Design review of the part built by this model. Coordinates are the model's own, in mm. Give positions to 0.01 mm unless a question says otherwise; leave off trailing zeros. Write each loop counter-clockwise with the first axis right and the second up, starting at its lowest first coordinate (ties: lowest second). Pieces come first, ordered by that corner, then holes. Notation, with made-up numbers: M -15,-37.75 L 42,-37.75 A14 cw 42,-30.75 Z; hole C 2,47.25 d5. An arc over 180 degrees is marked long. Use one line per item in the form item = value. Start each with the question number.
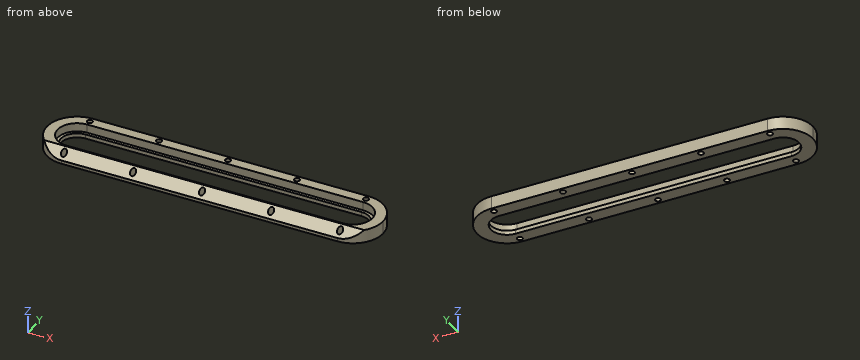
from build123d import *

# Parameters (mm, degrees)
SKETCH1_W              = 247.65
SKETCH1_H              = 44.45
BOSS_EXTRUDE1_DEPTH    = 9.525
CUT_EXTRUDE1_DEPTH     = 6.35
CUT_EXTRUDE3_DEPTH     = 126.963898598
CUT_EXTRUDE2_DEPTH     = 127.163809688
F_10_32_TAPPED_HOLE1_D = 4.0386
CHAMFER2_SIZE          = 6.985


with BuildPart() as part:
    # Sketch1 → Boss-Extrude1 (new body)
    with BuildSketch(Plane.XY):
        Rectangle(SKETCH1_W, SKETCH1_H)
    extrude(amount=BOSS_EXTRUDE1_DEPTH)

    # Sketch2 → Cut-Extrude1 (cut)
    with BuildSketch(Plane.XY.offset(9.525)):
        with BuildLine():
            Line((101.6, -14.351), (-101.6, -14.351))
            ThreePointArc((-101.6, -14.351), (-115.951, 0), (-101.6, 14.351))
            Line((-101.6, 14.351), (101.6, 14.351))
            ThreePointArc((101.6, 14.351), (115.951, 0), (101.6, -14.351))
        make_face()
    extrude(amount=-CUT_EXTRUDE1_DEPTH, mode=Mode.SUBTRACT)

    # Sketch14 → Cut-Extrude3 (cut, through all)
    with BuildSketch(Plane.XY.offset(3.175)):
        with BuildLine():
            Line((101.6, 11.96975), (-101.6, 11.96975))
            ThreePointArc((-101.6, 11.96975), (-113.56975, 0), (-101.6, -11.96975))
            Line((-101.6, -11.96975), (101.6, -11.96975))
            ThreePointArc((101.6, -11.96975), (113.56975, 0), (101.6, 11.96975))
        make_face()
    extrude(amount=-CUT_EXTRUDE3_DEPTH, mode=Mode.SUBTRACT)

    # Sketch3 → Cut-Extrude2 (cut, through all)
    with BuildSketch(Plane.XY.offset(9.525)):
        with BuildLine():
            ThreePointArc((-123.825, -1.74e-07), (-117.315448274, 15.71544815), (-101.6, 22.225))
            Line((-101.6, 22.225), (-123.825, 22.225))
            Line((-123.825, 22.225), (-123.825, -1.74e-07))
        make_face()
        with BuildLine():
            ThreePointArc((-101.6, -22.225), (-117.31544815, -15.715448274), (-123.825, -1.74e-07))
            Line((-123.825, -1.74e-07), (-123.825, -22.225))
            Line((-123.825, -22.225), (-101.6, -22.225))
        make_face()
        with BuildLine():
            Line((123.825, -22.225), (123.825, -6.4e-08))
            ThreePointArc((123.825, -6.4e-08), (117.315448189, -15.715448235), (101.6, -22.225))
            Line((101.6, -22.225), (123.825, -22.225))
        make_face()
        with BuildLine():
            Line((123.825, 22.225), (101.6, 22.225))
            ThreePointArc((101.6, 22.225), (117.315448235, 15.715448189), (123.825, -6.4e-08))
            Line((123.825, -6.4e-08), (123.825, 22.225))
        make_face()
    extrude(amount=-CUT_EXTRUDE2_DEPTH, mode=Mode.SUBTRACT)

    # #10-32 Tapped Hole1 (through all)
    with Locations(Plane.XY.offset(9.525)):
        with Locations((-101.6, 18.415), (-50.8, 18.415), (0, 18.415), (50.8, 18.415), (101.6, 18.415), (101.6, -18.415), (50.8, -18.415), (0, -18.415), (-50.8, -18.415), (-101.6, -18.415)):
            Hole(F_10_32_TAPPED_HOLE1_D / 2)

    # Chamfer2
    # the kernel refuses this chamfer: 6.985 mm, written as the material it takes off along each edge
    with BuildSketch(Plane(origin=(-119.563205671, -22.225, 9.525), x_dir=(0, 0.9996219169112968, 0.027495876610586303), z_dir=(1, 0, 0))) as chamfer2_piece_1:
        Polygon((CHAMFER2_SIZE * 0.999621916911, -CHAMFER2_SIZE * 0.0274958766106), (-CHAMFER2_SIZE * 0.0274958766106, -CHAMFER2_SIZE * 0.999621916911), (0, 0), align=None)
    extrude(amount=239.126411342, mode=Mode.SUBTRACT)


solid = part.part
1. We need section C-C (x = 108.5). State the section outline as (y, z) points (3 decimals).
2. We need section A-A (x = 15.5). State the section outline as (y, z) points (3 decimals).
3. We need section B-B (x = 50.8). State the section outline as (y, z) points (3 decimals).
4. Clearance check with flat-ended pins moving along their axes: pin 1 Ø1 at (y, z) = (2, 2.5) entering from +X; pin 2 Ø1 at (x, z) = (-69, 4) entering from -Y (3 decimals); pin 3 Ø4 at (y, z) = (-3.5, 7.5) entering from -X. State where each tip first meets the part, or that it passes through.
5. To check wall thickness, follow L1, parallel to Y at x = -50.8, z = 7.5 (3 decimals); L2, parallel to Y at x = 49.5, z = 6 (3 decimals); L3, parallel to X at y = 19, z = 2. State the ranges of each line that lie inside material, in increasing order.
Answer block:
q1.outline = M -21.127,0 L -9.781,0 L -9.781,3.175 L -12.583,3.175 L -12.583,9.525 L -15.24,9.525 L -21.127,3.638 Z; M 9.781,0 L 21.127,0 L 21.127,9.525 L 12.583,9.525 L 12.583,3.175 L 9.781,3.175 Z
q2.outline = M -22.225,0 L -11.97,0 L -11.97,3.175 L -14.351,3.175 L -14.351,9.525 L -15.24,9.525 L -22.225,2.54 Z; M 11.97,0 L 22.225,0 L 22.225,9.525 L 14.351,9.525 L 14.351,3.175 L 11.97,3.175 Z
q3.outline = M -22.225,0 L -20.434,0 L -20.434,4.331 L -22.225,2.54 Z; M -16.396,0 L -11.97,0 L -11.97,3.175 L -14.351,3.175 L -14.351,9.525 L -15.24,9.525 L -16.396,8.369 Z; M 11.97,0 L 16.396,0 L 16.396,9.525 L 14.351,9.525 L 14.351,3.175 L 11.97,3.175 Z; M 20.434,0 L 22.225,0 L 22.225,9.525 L 20.434,9.525 Z
q4.pin_1 = 123.77
q4.pin_2 = -21.265
q4.pin_3 = -123.77
q5.L1 = -16.396 to -14.351, 14.351 to 16.396, 20.434 to 22.225
q5.L2 = -16.87 to -14.351, 14.351 to 16.87, 19.96 to 22.225
q5.L3 = -113.13 to -103.53, -99.67 to -52.73, -48.87 to -1.93, 1.93 to 48.87, 52.73 to 99.67, 103.53 to 113.13
